Part model, mm, in its own coordinate system. Face numbers are marked on the shaded views. A direction names the side the tool comes from. Round coordinates to 2 decimals unless told otherwise and drop trailing zeros. Loops run counter-clockwise (first coordinate to the right, second up) from the corner with the lowest first, then second, coordinate; pieces in that order, holes last. Notation, with made-up numbers: M 28.5,74 L 32.5,74 A16 ccw 32.5,80 Z; hole C -15.5,50 d9. An arc over 180 degrees is marked long. Put each result on its own line as item: value. Start each with the question number.
1) Which spindle directions (+Z, -Z, +X, -X, +Y, -Y) get a long thin tool onto all of the face, cutting with end or side? Do the marked faces 1, 2 and 3. Say none if no direction does.
2) Drop flat-ended pins along their axis: pin 1 Ø19.5 at (x, z) = (-163.5, 14.5) entering from -Y; pin 2 Ø1 at (y, z) = (-78.5, 150.5) entering from +X. Give the stop position or say it passes through.
3) Slice it at A-A on y = -105.5. Give the cut face in (x, z), then the cut area to 3 significant figures.
4) Probe line 1 along Z through (x, y) = (-168, -40.5); line 2 along X through (y, z) = (-110, 106.5); line 3 along Z through (x, y) = (-58, -103). List the from-to ranges inside material, lowest first.
5) Slice it at B-B on z = 23. Give the cut face in (x, y), then the cut area to 3 significant figures.
6) Slice it at D-D on x = -56.5. Give the cut face in (y, z).
7) Pull direction X, two halves, no side cores. Call the marked faces 4, 5, 6 and 7: +X half, -X half, draft (parallel to the pull), parting line (faces both ways), or undercut.
8) Slice it at C-C on x = -174. Give the cut face in (y, z), then the cut area to 3 significant figures.
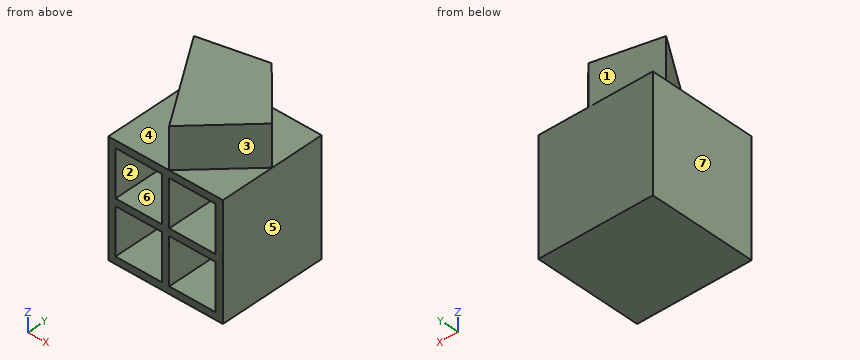
```python
from build123d import *

# Parameters (mm, degrees)
F0_W     = 160
F0_H     = 160
F0_W_2   = 65
F0_H_2   = 10
F0_W_3   = 10
F0_H_3   = 65
F1_DEPTH = 150
F2_W     = 10
F2_H     = 160
F3_DEPTH = 150
F5_DEPTH = 57


with BuildPart() as f1:
    # F0 (on Front) → F1 (new body)
    with BuildSketch(Plane.XZ):
        with Locations((-111.5596954525, 50.3307304141)):
            Rectangle(F0_W, F0_H)
        Polygon((-181.5596954525, 55.3307304141), (-181.5596954525, 120.3307304141), (-116.5596954525, 120.3307304141), (-106.5596954525, 120.3307304141), (-41.5596954525, 120.3307304141), (-41.5596954525, 55.3307304141), (-41.5596954525, 45.3307304141), (-41.5596954525, -19.6692695859), (-106.5596954525, -19.6692695859), (-116.5596954525, -19.6692695859), (-181.5596954525, -19.6692695859), (-181.5596954525, 45.3307304141), align=None, mode=Mode.SUBTRACT)
        with Locations((-149.0596954525, 50.3307304141)):
            Rectangle(F0_W_2, F0_H_2)
        with Locations((-111.5596954525, 87.8307304141)):
            Rectangle(F0_W_3, F0_H_3)
        with Locations((-74.0596954525, 50.3307304141)):
            Rectangle(F0_W_2, F0_H_2)
        with Locations((-111.5596954525, 12.8307304141)):
            Rectangle(F0_W_3, F0_H_3)
        with Locations((-111.5596954525, 50.3307304141)):
            Rectangle(F0_W_3, F0_H_2)
    extrude(amount=F1_DEPTH)

    # F2 (on face) → F3 (join)
    with BuildSketch(Plane.YZ.offset(-31.5596954525)):
        with Locations((-5, 50.3307304141)):
            Rectangle(F2_W, F2_H)
    extrude(amount=-F3_DEPTH)

    # F4 (on face) → F5 (join)
    with BuildSketch(Plane.XY.offset(130.3307304141)):
        Polygon((-101.4029532671, 0), (-191.5596954525, -20.1587285846), (-106.5589338541, -150), (-31.5596954525, -75), align=None)
    extrude(amount=F5_DEPTH)


solid = f1.part
```
Recorded:
1. face 1: +Z, -X, +Y
1. face 2: -Y
1. face 3: +Z, +X, -Y
2. pin 1: stops at y = -10
2. pin 2: stops at x = -34.56
3. outline: M -191.56,-29.67 L -31.56,-29.67 L -31.56,130.33 L -62.06,130.33 L -62.06,187.33 L -135.69,187.33 L -135.69,130.33 L -191.56,130.33 Z; hole M -181.56,-19.67 L -116.56,-19.67 L -116.56,45.33 L -181.56,45.33 Z; hole M -181.56,55.33 L -116.56,55.33 L -116.56,120.33 L -181.56,120.33 Z; hole M -106.56,-19.67 L -41.56,-19.67 L -41.56,45.33 L -106.56,45.33 Z; hole M -106.56,55.33 L -41.56,55.33 L -41.56,120.33 L -106.56,120.33 Z
3. area: 12,900 mm2
4. line 1: z = -29.67 to -19.67, 45.33 to 55.33, 120.33 to 187.33
4. line 2: x = -191.56 to -181.56, -116.56 to -106.56, -41.56 to -31.56
4. line 3: z = -29.67 to -19.67, 45.33 to 55.33, 120.33 to 130.33
5. outline: M -191.56,-150 L -181.56,-150 L -181.56,-10 L -116.56,-10 L -116.56,-150 L -106.56,-150 L -106.56,-10 L -41.56,-10 L -41.56,-150 L -31.56,-150 L -31.56,0 L -191.56,0 Z
5. area: 5,800 mm2
6. outline: M -150,-29.67 L 0,-29.67 L 0,130.33 L -48.22,130.33 L -48.22,187.33 L -99.94,187.33 L -99.94,130.33 L -150,130.33 L -150,120.33 L -10,120.33 L -10,55.33 L -150,55.33 L -150,45.33 L -10,45.33 L -10,-19.67 L -150,-19.67 Z
7. face 4: draft
7. face 5: +X half
7. face 6: undercut
7. face 7: -X half
8. outline: M -150,-29.67 L 0,-29.67 L 0,130.33 L -16.23,130.33 L -16.23,187.33 L -46.98,187.33 L -46.98,130.33 L -150,130.33 L -150,120.33 L -10,120.33 L -10,55.33 L -150,55.33 L -150,45.33 L -10,45.33 L -10,-19.67 L -150,-19.67 Z
8. area: 7,550 mm2
